Geometry: final body of the model. Coordinates: model frame, mm. A direction names the side the tool comes from. Give positions to 0.01 mm unless a question says otherwise; leave off trailing zeros. Write each loop counter-clockwise with the first axis right and the second up, starting at its lowest first coordinate (ties: lowest second). Pieces come first, ordered by that corner, then holes.
Q1. Pin query (flat end, axial travel): pin 1 (3.5 mm diameter, centred on x = -2.07, y = 5.5, fed in from -Z); pin 2 (1.5 mm diameter, centred on x = 6, y = 1, fed in from -Z); pin 3 (16 mm diameter, centred on x = 12.93, z = -1.72, fed in from +Y). Return the tip coordinate at first contact, or that it passes through.
Q2. Draft query along Z for faces 4 (the face through (9, -0.5, 2)), 5 (the face through (9, 5, 16.782)), 6 (the face through (12.9, -0.25, -14.72)). Return one class per face: pulls with the +Z half, pulls with the -Z half, needs draft (parallel to the pull), parting line crosses it, or undercut.
Q3. Line query: L1, parallel to Z at x = -10, y = 5.75; L2, parallel to Y at x = -0.5, z = 2.5. Output: solid intervals per line, ascending.
Q4. Cut plane D-D on y = 2.5. Return the cut outline in (x, z).
Q5. Reachability of faces 1 (the face through (9, 0, -6)), 2 (the face through (12.97, -0.25, -7.72)), 3 (the face through (-13.066, -0.3, -1.8)) from +Z, -Z, +X, -X, +Y, -Y: full face, straight path, thin tool, end or side. Return the list, or none.
Q6. Cut plane A-A on y = 5.5. Return the cut outline in (x, z).
Q7. Cut plane C-C on x = -10. Return the cut outline in (y, z), plus the area to 4 significant figures.
Q8. Cut plane B-B on z = 5. Return the cut outline in (x, y).
```python
from build123d import *

# Parameters (mm, degrees)
F0_W     = 45
F0_H     = 38
F1_DEPTH = 0.5
F2_W     = 45
F2_H     = 10
F2_R     = 1.5
F3_DEPTH = 0.5
F4_R     = 0.5
F5_R     = 5
F6_DEPTH = 25


with BuildPart() as f1:
    # F0 (on Front) → F1 (new body)
    with BuildSketch(Plane.XZ):
        with Locations((9.434236, -1.718442)):
            Rectangle(F0_W, F0_H)
    extrude(amount=F1_DEPTH)

    # F2 (on face) → F3 (join)
    with BuildSketch(Plane.XY.offset(17.281558)):
        with Locations((9.434236, 4.5)):
            Rectangle(F2_W, F2_H)
        with Locations((-2.065764, 5.5)):
            Circle(F2_R, mode=Mode.SUBTRACT)
        with Locations((25.934236, 5.5)):
            Circle(F2_R, mode=Mode.SUBTRACT)
    extrude(amount=-F3_DEPTH)

    # F4
    f4_edges = [f1.edges().sort_by_distance(p)[0] for p in [
        (9.434236, -0.5, 17.281558),
        (9.434236, 0, 16.781558),
    ]]
    fillet(f4_edges, radius=F4_R)

    # F5 (on face) → F6 (cut)
    with BuildSketch(Plane.XZ.offset(0.5)):
        with Locations((12.934236, -1.718442)):
            Circle(F5_R)
        with BuildLine():
            Line((14.434236, 5.781558), (14.434236, 9.781558))
            ThreePointArc((14.434236, 9.781558), (12.934236, 11.281558), (11.434236, 9.781558))
            Line((11.434236, 9.781558), (11.434236, 5.781558))
            ThreePointArc((11.434236, 5.781558), (12.934236, 4.281558), (14.434236, 5.781558))
        make_face()
        with BuildLine():
            Line((14.434236, -13.218442), (14.434236, -9.218442))
            ThreePointArc((14.434236, -9.218442), (12.934236, -7.718442), (11.434236, -9.218442))
            Line((11.434236, -9.218442), (11.434236, -13.218442))
            ThreePointArc((11.434236, -13.218442), (12.934236, -14.718442), (14.434236, -13.218442))
        make_face()
    extrude(amount=-F6_DEPTH, mode=Mode.SUBTRACT)


solid = f1.part
```
Data:
1. pin 1: stops at z = 16.78
1. pin 2: stops at z = 16.71
1. pin 3: stops at y = 0
2. face 4: needs draft
2. face 5: pulls with the -Z half
2. face 6: undercut
3. L1: z = 16.78 to 17.28
3. L2: y = -0.5 to 0
4. outline: (-13.07, 16.78) - (31.93, 16.78) - (31.93, 17.28) - (-13.07, 17.28) - close
5. face 1: -Z, +X, -X, +Y
5. face 2: +Y, -Y
5. face 3: +Z, -Z, -X, +Y, -Y
6. outline: (-13.07, 16.78) - (-3.57, 16.78) - (-3.57, 17.28) - (-13.07, 17.28) - close; (-0.57, 16.78) - (24.43, 16.78) - (24.43, 17.28) - (-0.57, 17.28) - close; (27.43, 16.78) - (31.93, 16.78) - (31.93, 17.28) - (27.43, 17.28) - close
7. outline: (-0.5, -20.72) - (0, -20.72) - (0, 16.28) arc R0.5 cw to (0.5, 16.78) - (9.5, 16.78) - (9.5, 17.28) - (0, 17.28) arc R0.5 ccw to (-0.5, 16.78) - close
7. area: 23.75 mm2
8. outline: (-13.07, -0.5) - (11.65, -0.5) - (11.65, 0) - (-13.07, 0) - close; (14.21, -0.5) - (31.93, -0.5) - (31.93, 0) - (14.21, 0) - close
